The listing builds one solid part. Answer for the finished solid, in the listing's coordinates (mm). Face numbers are marked on the shaded views. A direction names the side the tool comes from. Round coordinates to 2 decimals unless told otherwise and drop trailing zeros. Write each loop counter-clockwise with the first axis right and the second up, starting at its lowest first coordinate (ties: lowest second). Pieces come first, ordered by that corner, then holes. Notation, with made-up numbers: (-15, -35) - (13, -35) arc R14 ccw to (13, -20) - close; hole circle Ø5 at (-4, 48). An arc over 180 degrees is marked (long way). Answer in a Markdown table with one row per item.
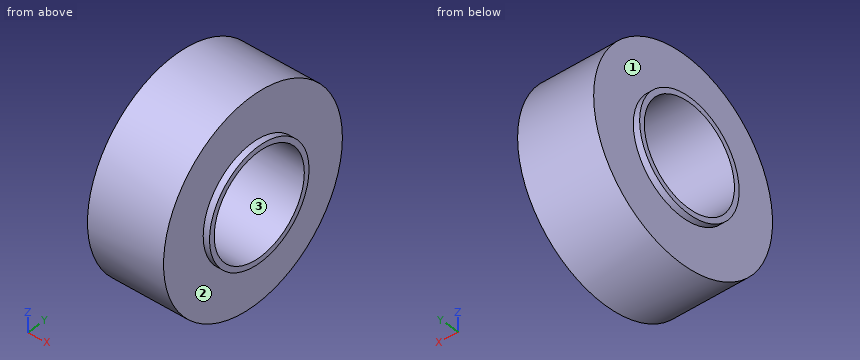
from build123d import *

# Parameters (mm, degrees)
F0_R     = 6.35
F0_R_2   = 3.2004
F1_DEPTH = 2.38125
F2_R     = 3.535
F2_R_2   = 3.2004
F3_DEPTH = 2.775


# Not quite as in the source:
# - a length typed as a fraction of an inch, garbled in the dataset ("3 / 203.2 mm" for 3/8 in), is restored


with BuildPart() as f1:
    # F0 (on Right) → F1 (new body, symmetric)
    with BuildSketch(Plane.YZ):
        Circle(F0_R)
        Circle(F0_R_2, mode=Mode.SUBTRACT)
    extrude(amount=F1_DEPTH, both=True)

    # F2 (on Right) → F3 (join, symmetric)
    with BuildSketch(Plane.YZ):
        Circle(F2_R)
        Circle(F2_R_2, mode=Mode.SUBTRACT)
    extrude(amount=F3_DEPTH, both=True)


solid = f1.part
(1) For the marked faces 1, 2 and 3, determine the directions among +Z, -Z, +X, -X, +Y, -Y from which every point of the face is accessible in a straight line to the end or side of a thin tool.
Checked values:
| item | result |
|---|---|
| face 1 | -X |
| face 2 | +X |
| face 3 | +X, -X |
(2) Section A-A (z = 0) is taken. Give the vertices of the cut face in (x, y) (3 decimals), and give its area (3 significant figures).
Checked values:
| item | result |
|---|---|
| outline | (-2.775, -3.535) - (-2.381, -3.535) - (-2.381, -6.35) - (2.381, -6.35) - (2.381, -3.535) - (2.775, -3.535) - (2.775, -3.2) - (-2.775, -3.2) - close; (-2.775, 3.2) - (2.775, 3.2) - (2.775, 3.535) - (2.381, 3.535) - (2.381, 6.35) - (-2.381, 6.35) - (-2.381, 3.535) - (-2.775, 3.535) - close |
| area | 30.5 mm2 |
(3) Flat-ended cylindrical pins translate along their axes: pin 1 (1.5 mm diameter, centred on x = 1.5, z = -3.5, fed in from +Y); pin 2 (2 mm diameter, centred on y = 4.5, z = -1, fed in from +X). Find the tip coordinate at first contact, or state that the pin passes through.
Checked values:
| item | result |
|---|---|
| pin 1 | stops at y = 5.72 |
| pin 2 | stops at x = 2.38 |
(4) Find the intervals of material crossed by line 1 (Z direction, x = -0.4, y = 0); line 2 (X direction, y = 4.25, z = -0.5); line 3 (Z direction, x = -1.2, y = 1.75), in increasing order.
Checked values:
| item | result |
|---|---|
| line 1 | z = -6.35 to -3.2, 3.2 to 6.35 |
| line 2 | x = -2.38 to 2.38 |
| line 3 | z = -6.1 to -2.68, 2.68 to 6.1 |
(5) Section C-C (x = 0.25) is taken. Give the vertices of the cut face in (y, z).
Checked values:
| item | result |
|---|---|
| outline | circle Ø12.7 at (0, 0); hole circle Ø6.4 at (0, 0) |
(6) Section D-D (y = -4) is taken. Give the vertices of the cut face in (x, z), and give its area (3 significant figures).
Checked values:
| item | result |
|---|---|
| outline | (-2.38, -4.93) - (2.38, -4.93) - (2.38, 4.93) - (-2.38, 4.93) - close |
| area | 47.0 mm2 |
